from build123d import *

# Parameters (mm, degrees)
F0_R     = 25
F0_R_2   = 5
F0_R_3   = 3
F0_R_4   = 3.5
F1_DEPTH = 28
F2_T     = -4
F3_DEPTH = 25
F4_R     = 25
F5_DEPTH = 2


# Not quite as in the source:
# - a feature names something its author has since deleted; it is built from what else it names


with BuildPart() as f1:
    # F0 (on Top) → F1 (new body)
    with BuildSketch(Plane.XY):
        Circle(F0_R)
        with Locations((-12.990381, -7.5)):
            Circle(F0_R_2, mode=Mode.SUBTRACT)
        with Locations((0, -15)):
            Circle(F0_R_3, mode=Mode.SUBTRACT)
        with Locations((12.990381, -7.5)):
            Circle(F0_R_2, mode=Mode.SUBTRACT)
        with Locations((-12.990381, 7.5)):
            Circle(F0_R_3, mode=Mode.SUBTRACT)
        Circle(F0_R_4, mode=Mode.SUBTRACT)
        with Locations((12.990381, 7.5)):
            Circle(F0_R_3, mode=Mode.SUBTRACT)
        with Locations((0, 15)):
            Circle(F0_R_2, mode=Mode.SUBTRACT)
        Circle(F0_R_4)
        with Locations((-12.990381, 7.5)):
            Circle(F0_R_3)
        with Locations((12.990381, 7.5)):
            Circle(F0_R_3)
        with Locations((0, -15)):
            Circle(F0_R_3)
    extrude(amount=F1_DEPTH)

    # F2
    f2_openings = [f1.faces().sort_by_distance(p)[0] for p in [
        (0, 0, 28),
    ]]
    offset(amount=F2_T, openings=f2_openings)

    # F0 (on Top) → F3 (cut)
    with BuildSketch(Plane.XY):
        with Locations((-12.990381, 7.5)):
            Circle(F0_R_3)
        Circle(F0_R_4)
        with Locations((12.990381, 7.5)):
            Circle(F0_R_3)
        with Locations((0, -15)):
            Circle(F0_R_3)
    extrude(amount=F3_DEPTH, mode=Mode.SUBTRACT)

    # F4 (on face) → F5 (join)
    with BuildSketch(Plane.XY.offset(28)):
        Circle(F4_R)
        with BuildLine():
            ThreePointArc((-20.78461, -3), (-18.186533, 10.5), (-7.794229, 19.5))
            ThreePointArc((-7.794229, 19.5), (0, 6), (7.794229, 19.5))
            ThreePointArc((7.794229, 19.5), (18.186533, 10.5), (20.78461, -3))
            ThreePointArc((20.78461, -3), (5.196152, -3), (12.990381, -16.5))
            ThreePointArc((12.990381, -16.5), (0, -21), (-12.990381, -16.5))
            ThreePointArc((-12.990381, -16.5), (-5.196152, -3), (-20.78461, -3))
        make_face(mode=Mode.SUBTRACT)
    extrude(amount=F5_DEPTH)


solid = f1.part
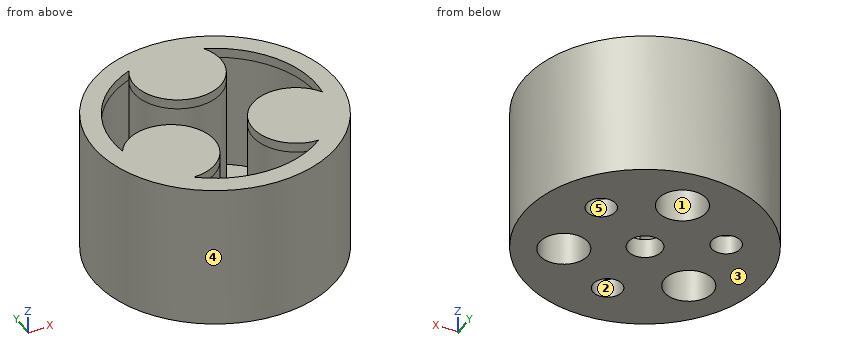
Build history of the part. All positions in model axes, mm. Face numbers are marked on the shaded views. A direction names the side the tool comes from. Round coordinates to 2 decimals unless told otherwise and drop trailing zeros. Write each loop counter-clockwise with the first axis right and the second up, starting at its lowest first coordinate (ties: lowest second). Pieces come first, ordered by that corner, then holes. Notation, with made-up numbers: (-32.5, -7) -> (-16.5, -7) arc R21 cw to (-16.5, 7) -> close; hole circle Ø5 at (5, 3.25). An arc over 180 degrees is marked (long way). Write item = value, one per line.
(1) Tool access for the marked faces 1 and 2: list every direction of +Z, -Z, +X, -X, +Y, -Y with a clear straight run to the whole face (end or side of a thin tool).
Answer:
face_1 = -Z
face_2 = +Z, -Z
(2) Flat gauge pins, fed straight in: pin 1 (4 mm diameter, centred on x = 3, z = 23, fed in from +Y); pin 2 (8 mm diameter, centred on x = -2.5, y = -15.5, fed in from +Z); pin 3 (1 mm diameter, centred on x = -14, z = 4, fed in from +Y). Where does each tip first touch, or does it go through?
Answer:
pin_1 = 24.98
pin_2 = 4
pin_3 = 21.04
(3) Two-plate mould, pull along Y, no slides. Class the marked faces 3, 4 and 5: pulls with the +Y half, pulls with the -Y half, needs draft (parallel to the pull), parting line crosses it, or undercut.
Answer:
face_3 = needs draft
face_4 = parting line crosses it
face_5 = undercut
(4) Band-saw the part on A-A (x = 0). Give the cut face in (y, z).
Answer:
outline = (-25, 0) -> (-18, 0) -> (-18, 4) -> (-21, 4) -> (-21, 30) -> (-25, 30) -> close; (-12, 0) -> (-3.5, 0) -> (-3.5, 4) -> (-12, 4) -> close; (3.5, 0) -> (10, 0) -> (10, 28) -> (20, 28) -> (20, 0) -> (25, 0) -> (25, 30) -> (6, 30) -> (6, 4) -> (3.5, 4) -> close
(5) Band-saw the part on B-B (y = -15). Give the cut face in (x, z).
Answer:
outline = (-20, 0) -> (-3, 0) -> (-3, 4) -> (-8.02, 4) -> (-8.02, 30) -> (-20, 30) -> close; (3, 0) -> (20, 0) -> (20, 30) -> (8.02, 30) -> (8.02, 4) -> (3, 4) -> close
(6) Band-saw the part on C-C (z = 18.25). Give the cut face in (x, y), then the cut area to 3 significant figures.
Answer:
outline = circle Ø50 at (0, 0); hole (-20.78, -3) arc R9 cw (long way) to (-12.99, -16.5) arc R21 ccw to (12.99, -16.5) arc R9 cw (long way) to (20.78, -3) arc R21 ccw to (7.79, 19.5) arc R9 cw (long way) to (-7.79, 19.5) arc R21 ccw to start; hole circle Ø10 at (-12.99, -7.5); hole circle Ø10 at (0, 15); hole circle Ø10 at (12.99, -7.5)
area = 1,000 mm2
(7) Band-saw the part on D-D (y = 7.5). Give the cut face in (x, z).
Answer:
outline = (-23.85, 0) -> (-15.99, 0) -> (-15.99, 4) -> (-19.62, 4) -> (-19.62, 30) -> (-23.85, 30) -> close; (-9.99, 0) -> (9.99, 0) -> (9.99, 4) -> (4.97, 4) -> (4.97, 30) -> (-4.97, 30) -> (-4.97, 4) -> (-9.99, 4) -> close; (15.99, 0) -> (23.85, 0) -> (23.85, 30) -> (19.62, 30) -> (19.62, 4) -> (15.99, 4) -> close
(8) Probe L1, parallel to Y at x = 0, z = 2.7; L2, parallel to X at y = -9, z = 14.75; L3, parallel to X at y = 19, z = 27.5. List the from-to ranges inside material, lowest first.
Answer:
L1 = -25 to -18, -12 to -3.5, 3.5 to 10, 20 to 25
L2 = -23.32 to -17.76, -8.22 to -4.12, 4.12 to 8.22, 17.76 to 23.32
L3 = -16.25 to -8.94, -8.06 to -3, 3 to 8.06, 8.94 to 16.25
